CAD build for the part. Positions are in the model's coordinates, mm. A direction names the side the tool comes from. Round coordinates to 2 decimals unless told otherwise and drop trailing zeros. Answer in a Markdown table with one row per item.
```python
from build123d import *

# Parameters (mm, degrees)
RESSALTO_EXTRUS_O1_DEPTH                = 75
CORTE_EXTRUS_O1_DEPTH                   = 70
CORTE_EXTRUS_O1_DEPTH_BACK              = 70
ESBO_O2_W                               = 63.930126489
ESBO_O2_H                               = 45
ESBO_O3_R                               = 12.5
CORTE_EXTRUS_O2_DEPTH                   = 103.728030149
FILETE1_R                               = 3
BROCA_DE_ROSQUEAR_PARA_TARRAXA_DE_M61_D = 5


with BuildPart() as part:
    # Esboço1 → Ressalto-extrusão1 (new body)
    with BuildSketch(Plane.XY):
        with BuildLine():
            ThreePointArc((55.829329515, 28.095123526), (60.733716713, 14.420104299), (62.5, 0))
            ThreePointArc((62.5, 0), (60.733716713, -14.420104299), (55.829329515, -28.095123526))
            add(Edge.make_bspline(
                [(28.676911595, -21.588340477), (43.861491247, -18.534041768), (55.829329515, -28.095123526)],
                knots=[0, 0, 0, 1, 1, 1], degree=2))
            add(Edge.make_bspline(
                [(-29.594432007, -31.676619774), (-9.724198858, -33.439461038), (9.873119669, -26.770904045), (28.676911595, -21.588340477)],
                knots=[0, 0, 0, 0, 1, 1, 1, 1], degree=3))
            add(Edge.make_bspline(
                [(-56.430126489, 0), (-56.804873179, -15.057396007), (-45.200173771, -30.412276657), (-29.594432007, -31.676619774)],
                knots=[0, 0, 0, 0, 1, 1, 1, 1], degree=3))
            add(Edge.make_bspline(
                [(-56.430126489, 0), (-56.804873179, 15.057396007), (-45.200173771, 30.412276657), (-29.594432007, 31.676619774)],
                knots=[0, 0, 0, 0, 1, 1, 1, 1], degree=3))
            add(Edge.make_bspline(
                [(-29.594432007, 31.676619774), (-9.724198858, 33.439461038), (9.873119669, 26.770904045), (28.676911595, 21.588340477)],
                knots=[0, 0, 0, 0, 1, 1, 1, 1], degree=3))
            add(Edge.make_bspline(
                [(28.676911595, 21.588340477), (43.861491247, 18.534041768), (55.829329515, 28.095123526)],
                knots=[0, 0, 0, 1, 1, 1], degree=2))
        make_face()
    extrude(amount=RESSALTO_EXTRUS_O1_DEPTH)

    # Esboço2 → Corte-extrusão1 (cut, two sides: drawn at the far end of the back side and taken through both)
    with BuildSketch(Plane(origin=(0, 0, 0), x_dir=(1, 0, 0), z_dir=(0, 1, 0)).offset(-CORTE_EXTRUS_O1_DEPTH_BACK)):
        with Locations((5.534936755, -37.5)):
            Rectangle(ESBO_O2_W, ESBO_O2_H)
    extrude(amount=CORTE_EXTRUS_O1_DEPTH + CORTE_EXTRUS_O1_DEPTH_BACK, mode=Mode.SUBTRACT)

    # Esboço3 → Corte-extrusão2 (cut, through all)
    with BuildSketch(Plane.XY.offset(75)):
        Circle(ESBO_O3_R)
    extrude(amount=-CORTE_EXTRUS_O2_DEPTH, mode=Mode.SUBTRACT)

    # Filete1
    filete1_edges = [part.edges().sort_by_distance(p)[0] for p in [
        (37.5, 0, 60),
        (37.5, 0, 15),
        (-26.430126489, 0, 60),
        (-26.430126489, 0, 15),
    ]]
    fillet(filete1_edges, radius=FILETE1_R)

    # Broca de rosquear para tarraxa de M61 (through all)
    with Locations(Plane.XY.offset(75)):
        with Locations((-6.180339887, 19.021130326), (16.180339887, 11.755705046), (16.180339888, -11.755705046), (-6.180339887, -19.021130326), (-20, 0)):
            Hole(BROCA_DE_ROSQUEAR_PARA_TARRAXA_DE_M61_D / 2)


solid = part.part
```
Q1. 3-axis set-ups, long thin cutter, end or side, ignore diameter. For faces 3 (the flat face through (-26.43, 0, 38)), 4 (the cylindrical face through (15.027, -13.974, 7.395)): which of +Z, -Z, +X, -X, +Y, -Y reach the whole face in a straight line?
Computed:
| item | result |
|---|---|
| face 3 | +Y, -Y |
| face 4 | +Z, -Z |
Q2. Pull direction Z, two halves, no side cores. Call faces 1 (the cylindrical face through (-7.33, 16.8, 67.4)), 2 (the cylindrical face through (-25.53, 0.45, 59.14)): released by +Z, released by -Z, zero draft, split by the parting line, or undercut.
Computed:
| item | result |
|---|---|
| face 1 | zero draft |
| face 2 | undercut |
Q3. Drill centre lines: line 1 (Z direction, x = 21.5, y = -7); line 2 (Y direction, x = -20, z = 69.25); line 3 (X direction, y = 1, z = 65). Where is each one in solid material? Low to high.
Computed:
| item | result |
|---|---|
| line 1 | z = 0 to 15, 60 to 75 |
| line 2 | y = -31.91 to -2.5, 2.5 to 31.91 |
| line 3 | x = -56.44 to -22.29, -17.71 to -12.46, 12.46 to 62.48 |
Q4. Saw through at A-A on x = -20. Count the separate pieces of the cut face and the enclosed holes in it, then the cut area to 3 significant figures.
Computed:
| item | result |
|---|---|
| separate pieces | 4 |
| enclosed holes | 0 |
| area | 1,760 mm2 |
Q5. Flat gauge pins, fed straight in: pin 1 (22.5 mm diameter, centred on x = 0, y = 0, fed in from -Z); pin 2 (4 mm diameter, centred on x = -37, z = 22.5, fed in from +Y); pin 3 (5 mm diameter, centred on y = -23, z = 62, fed in from +X); pin 4 (2 mm diameter, centred on y = 15.5, z = 61.5, fed in from +X). Where does each tip first touch, or does it go through?
Computed:
| item | result |
|---|---|
| pin 1 | passes through |
| pin 2 | stops at y = 30.65 |
| pin 3 | stops at x = 58.98 |
| pin 4 | stops at x = 60.71 |
